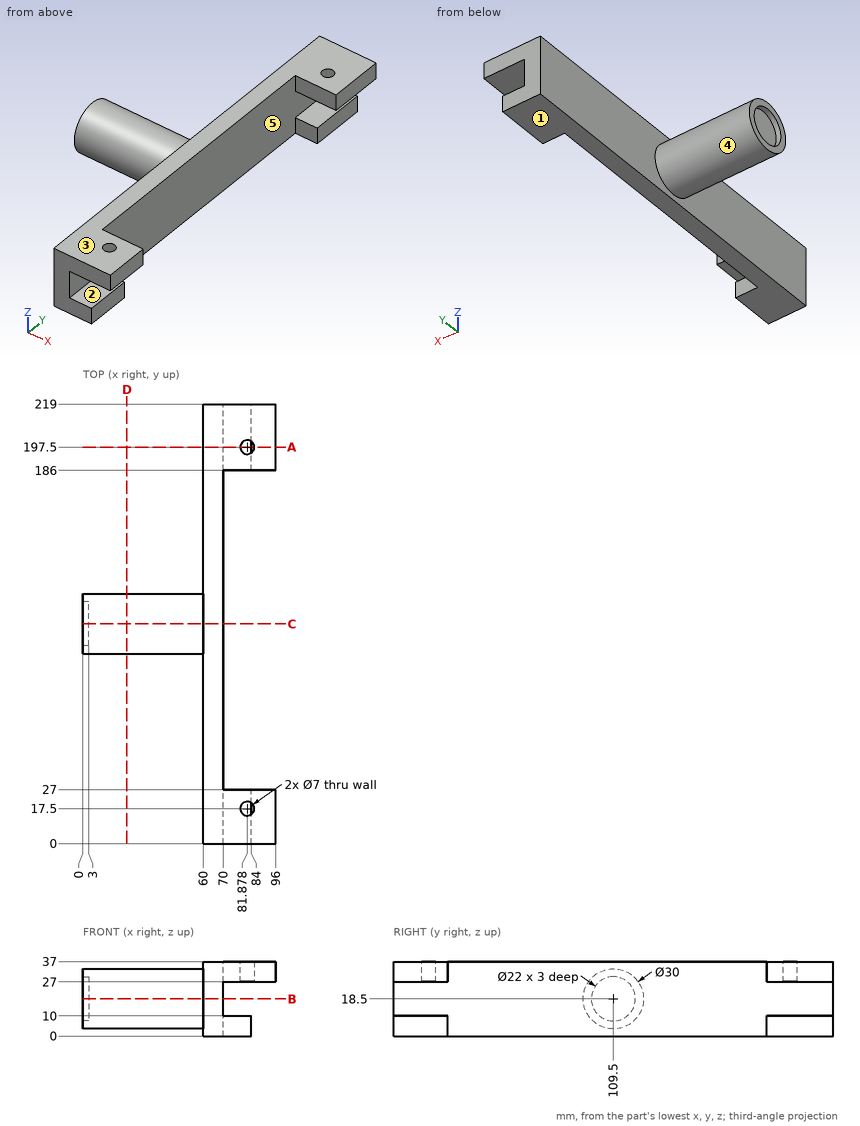
Answer from the drawing. Dimensions are ordinates in mm from the lowest x, y and z of the part. A direction names the side the tool comes from. Give positions to 0.01 mm unless a question says otherwise; leave off trailing zeros. Loops run counter-clockwise (first coordinate to the right, second up) from the corner with the lowest first, then second, coordinate; pieces in that order, holes last.
Item 1: The part is cut by section B-B (z = 18.5). Write down the section's boundary in (x, y).
Item 2: The part is cut by section A-A (y = 197.5). Write down the section's boundary in (x, z).
Item 3: The mould has two halves that part along Y. Classify the marked faces 3, 4 and 5: released by +Y, released by -Y, zero draft, split by the parting line, or undercut.
Item 4: Each of these flat-tipped pins is pushed along its axis until it touches: pin 1 Ø11 at (x, z) = (78.5, 6.5) entering from -Y; pin 2 Ø6 at (y, z) = (51, 13.5) entering from -X; pin 3 Ø3 at (y, z) = (209, 5) entering from +X; pin 4 Ø12 at (x, z) = (30.5, 18) entering from -Y. Where does it stop, or does it pass through?
Item 5: For the marked faces 1 and 2, determine the directions among +Z, -Z, +X, -X, +Y, -Y from which every point of the face is accessible in a straight line to the end or side of a thin tool.
Item 6: The part is cut by section C-C (y = 109.5). Write down the section's boundary in (x, z), and give its area (3 significant figures).
Item 7: Find the intervals of material crossed by line 1 along Y through (x, z) = (79.5, 2.5); line 2 along X through (y, z) = (197.5, 30.75); line 3 along X through (y, z) = (17, 29), in increasing order.
Item 8: The part is cut by section D-D (x = 22). Write down the section's boundary in (y, z), and give its area (3 significant figures).
Taken from the geometry:
1. outline: (0, 94.5) - (60, 94.5) - (60, 0) - (70, 0) - (70, 219) - (60, 219) - (60, 124.5) - (0, 124.5) - (0, 120.5) - (3, 120.5) - (3, 98.5) - (0, 98.5) - close
2. outline: (60, 0) - (84, 0) - (84, 10) - (70, 10) - (70, 27) - (78.38, 27) - (78.38, 37) - (60, 37) - close; (85.38, 27) - (96, 27) - (96, 37) - (85.38, 37) - close
3. face 3: zero draft
3. face 4: split by the parting line
3. face 5: undercut
4. pin 1: stops at y = 0
4. pin 2: stops at x = 60
4. pin 3: stops at x = 84
4. pin 4: stops at y = 94.5
5. face 1: -Z, +X, -X, +Y, -Y
5. face 2: +X, +Y, -Y
6. outline: (0, 3.5) - (60, 3.5) - (60, 0) - (70, 0) - (70, 37) - (60, 37) - (60, 33.5) - (0, 33.5) - (0, 29.5) - (3, 29.5) - (3, 7.5) - (0, 7.5) - close
6. area: 2,100 mm2
7. line 1: y = 0 to 27, 186 to 219
7. line 2: x = 60 to 78.38, 85.38 to 96
7. line 3: x = 60 to 78.41, 85.34 to 96
8. outline: circle Ø30 at (109.5, 18.5)
8. area: 707 mm2
